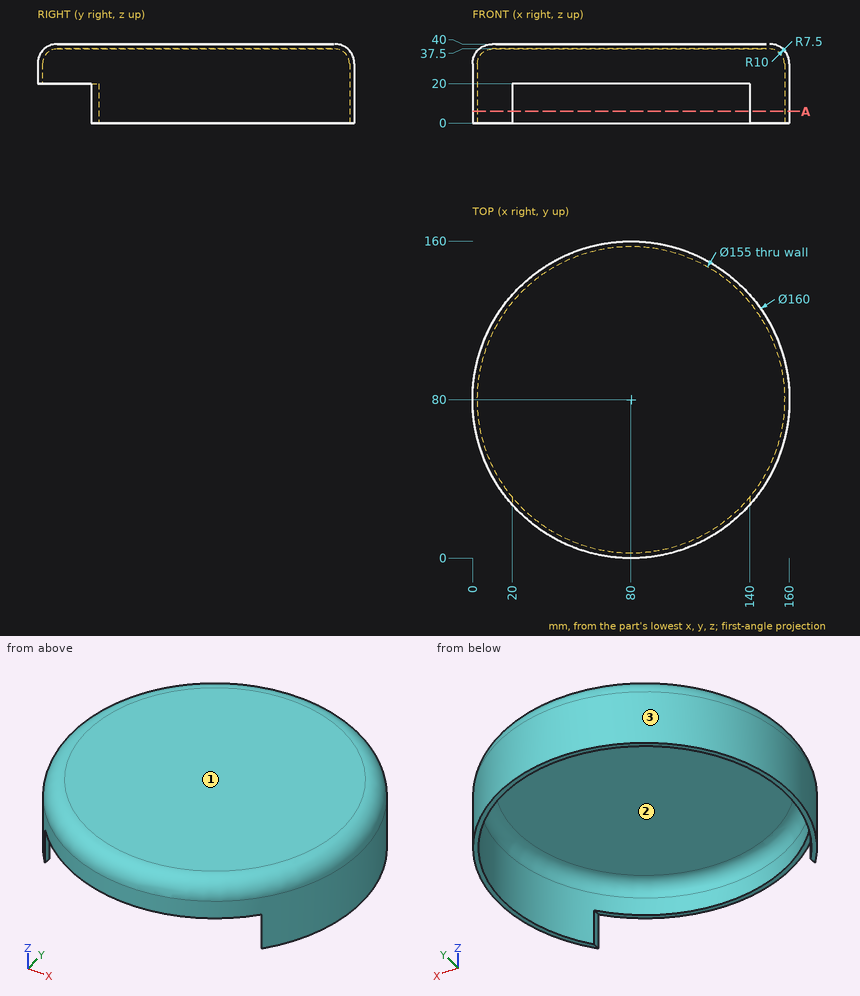
For this review, use the dimensioned drawing (mm, ordinates from the lowest corner) and the shaded views. Coordinates: 2 decimals unless noted, no trailing zeros. Loops run counter-clockwise (first coordinate to the right, second up) from the corner with the lowest first, then second, coordinate; pieces in that order, holes last. Notation, with made-up numbers: (33, 66) -> (53, 66) arc R38 cw to (53, 105) -> close; hole circle Ø7 at (83.25, -3.75). An arc over 180 degrees is marked (long way). Use a Markdown table: item, result. Add a question column.
1. To check wall thickness, follow line 1 (X direction, y = 80, z = 21.5); line 2 (Z direction, x = 35, y = 87.5); line 3 (Y direction, x = 12.5, z = 20). State the ranges of each line that lie inside material, in increasing order.
2. Add section A-A on z = 6. Write out the cut boundary in (x, y), plus the area to 3 significant figures.
3. Clearance check with flat-ended pins moving along their axes: pin 1 Ø25 at (x, y) = (98, 18.5) entering from -Z; pin 2 Ø1 at (x, y) = (90, 28.5) entering from -Z; pin 3 Ø1.2 at (y, z) = (28, 5) entering from +X. State where each tip first meets the part, or that it passes through.
4. Draft analysis for pull direction X (two halves, no side actions). For the marked faces 1, 2 and 3, state which applies: pulls with the +X half, pulls with the -X half, needs draft (parallel to the pull), parting line crosses it, or undercut.
Returned:
| question | item | result |
|---|---|---|
| 1 | line 1 | x = 0 to 2.5, 157.5 to 160 |
| 1 | line 2 | z = 37.5 to 40 |
| 1 | line 3 | y = 37.06 to 41.92, 118.08 to 122.94 |
| 2 | outline | (20, 27.08) -> (20, 30.95) arc R77.5 cw (long way) to (140, 30.95) -> (140, 27.08) arc R80 ccw (long way) to start |
| 2 | area | 896 mm² |
| 3 | pin 1 | stops at z = 33.6 |
| 3 | pin 2 | stops at z = 37.5 |
| 3 | pin 3 | stops at x = 141.3 |
| 4 | face 1 | needs draft |
| 4 | face 2 | undercut |
| 4 | face 3 | parting line crosses it |
